Verification items for this drawing (mm, ordinates from the low corner). Give positions to 0.01 mm unless a question says otherwise; leave off trailing zeros. Order: outer loops, then holes, each group sorted by start corner. A loop starts at its lowest first (then second) coordinate and runs counter-clockwise, first axis right, second up.
(1) Scan line: L1, parallel to Z at x = 61, y = 113.5. Record every from-to range of solid material in increasing order.
(2) Sectioned sample at C-C on y = 88. Record the cut outline in (x, z).
(3) Sectioned sample at B-B on y = 38.5. Record the cut outline in (x, z).
(4) Sectioned sample at A-A on x = 100. Record the cut outline in (y, z).
(5) Gauge pin test, flat end, axial feed: pin 1 (12 mm diameter, centred on x = 59.5, y = 121, fed in from +Z). Record the tip position at first contact, or that the pin passes through.
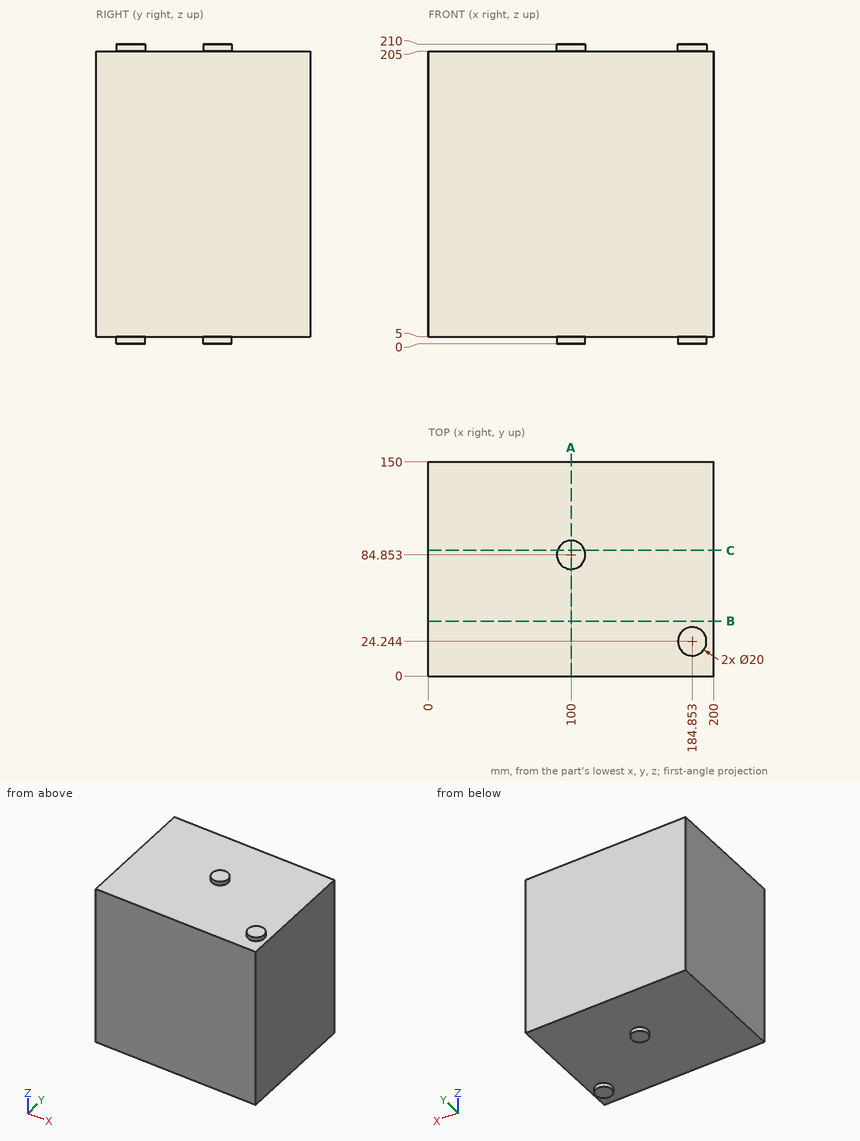
Ans:
1. L1: z = 5 to 205
2. outline: (0, 5) - (90.51, 5) - (90.51, 0) - (109.49, 0) - (109.49, 5) - (200, 5) - (200, 205) - (109.49, 205) - (109.49, 210) - (90.51, 210) - (90.51, 205) - (0, 205) - close
3. outline: (0, 5) - (200, 5) - (200, 205) - (0, 205) - close
4. outline: (0, 5) - (74.85, 5) - (74.85, 0) - (94.85, 0) - (94.85, 5) - (150, 5) - (150, 205) - (94.85, 205) - (94.85, 210) - (74.85, 210) - (74.85, 205) - (0, 205) - close
5. pin 1: stops at z = 205
